Can you work these out from the model? Positions are in its coordinate system, mm. Face numbers are marked on the shaded views. A direction names the side the tool comes from. Give positions to 0.01 mm unless a question says otherwise; leave off trailing zeros. Order: outer loops, then holes, each group sorted by start corner. A loop starts at its lowest first (then second) coordinate and runs counter-clockwise, first axis right, second up. Notation, with made-up numbers: M 84,-1 L 111,-1 A21 ccw 111,31 Z; hole C 41,15.5 d10. An arc over 180 degrees is marked long. Write each question's results on one line, items separated by ' | '.
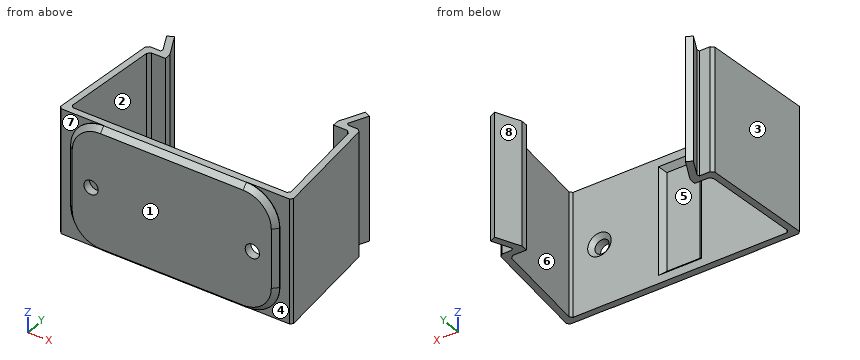
from build123d import *
from OCP.BRepFilletAPI import BRepFilletAPI_MakeChamfer

# Parameters (mm, degrees)
BOSS_EXTRUDE1_DEPTH                               = 38
SKETCH5_W                                         = 63
SKETCH5_H                                         = 38
BOSS_EXTRUDE2_DEPTH                               = 1.6
SKETCH9_W                                         = 10
SKETCH9_H                                         = 30
CUT_EXTRUDE4_DEPTH                                = 1.5
CHAMFER4_SIZE                                     = 1.5
CHAMFER6_SIZE                                     = 0.8
CHAMFER6_SIZE2                                    = 0.738449877
CHAMFER7_SIZE                                     = 0.8
CHAMFER7_SIZE2                                    = 0.880050294
CHAMFER7_SIZE2_2                                  = 0.59857957
CSK_FOR_6_FLAT_HEAD_MACHINE_SCREW_100_D           = 4.3053
CSK_FOR_6_FLAT_HEAD_MACHINE_SCREW_100_DEPTH       = 3.6
CSK_FOR_6_FLAT_HEAD_MACHINE_SCREW_100_CSINK_D     = 7.0866
CSK_FOR_6_FLAT_HEAD_MACHINE_SCREW_100_CSINK_ANGLE = 100
FILLET1_R                                         = 10
CHAMFER10_SIZE                                    = 1.5


with BuildPart() as part:
    # Sketch1 → Boss-Extrude1 (new body)
    with BuildSketch(Plane.XY):
        Polygon((-32.16425811, 32.5), (-27.555232111, 32.5), (-30.546782223, 38.65618727), (-28.747926936, 39.530326652), (-25.331595762, 32.5), (-25.331595762, 30.5), (-30.331595762, 30.5), (-33, 0), (0, 0), (33, 0), (30.331595762, 30.5), (25.331595762, 30.5), (25.331595762, 32.5), (28.747926936, 39.530326652), (30.546782223, 38.65618727), (27.555232111, 32.5), (32.16425811, 32.5), (35.182617002, -2), (0, -2), (-35.182617002, -2), align=None)
    extrude(amount=BOSS_EXTRUDE1_DEPTH)

    # Sketch5 → Boss-Extrude2 (add)
    with BuildSketch(Plane.XZ.offset(2)):
        with Locations((0, 19)):
            Rectangle(SKETCH5_W, SKETCH5_H)
    extrude(amount=BOSS_EXTRUDE2_DEPTH)

    # Sketch9 → Cut-Extrude4 (cut)
    with BuildSketch(Plane(origin=(0, 0, 0), x_dir=(1, 0, 0), z_dir=(0, 1, 0))):
        with Locations((0, -19)):
            Rectangle(SKETCH9_W, SKETCH9_H)
    extrude(amount=-CUT_EXTRUDE4_DEPTH, mode=Mode.SUBTRACT)

    # Chamfer4
    chamfer4_edges = [part.edges().sort_by_distance(p)[0] for p in [
        (0, 0, 34),
        (-5, 0, 19),
        (0, 0, 4),
        (5, 0, 19),
    ]]
    chamfer(chamfer4_edges, length=CHAMFER4_SIZE - 0.0001)  # a hair under: the kernel refuses the full size

    # Chamfer6: one chamfer whose edges measure the first distance from different faces: ONE call of the kernel's chamfer builder (chamfer() names one face for all edges)
    chamfer6_edges_1 = [part.edges().sort_by_distance(p)[0] for p in [
        (-33, 0, 19),
    ]]
    chamfer6_side_1 = [part.faces().sort_by_distance(p)[0] for p in [
        (0, 0, 36.261477311),
    ]]
    chamfer6_edges_2 = [part.edges().sort_by_distance(p)[0] for p in [
        (33, 0, 19),
    ]]
    chamfer6_side_2 = [part.faces().sort_by_distance(p)[0] for p in [
        (31.665797881, 15.25, 19),
    ]]
    chamfer6_edges_3 = [part.edges().sort_by_distance(p)[0] for p in [
        (35.182617002, -2, 19),
    ]]
    chamfer6_side_3 = [part.faces().sort_by_distance(p)[0] for p in [
        (33.341308501, -2, 19),
    ]]
    chamfer6_edges_4 = [part.edges().sort_by_distance(p)[0] for p in [
        (-35.182617002, -2, 19),
    ]]
    chamfer6_side_4 = [part.faces().sort_by_distance(p)[0] for p in [
        (-33.673437556, 15.25, 19),
    ]]
    chamfer6 = BRepFilletAPI_MakeChamfer(part.part.solid().wrapped)
    for e in chamfer6_edges_1:
        chamfer6.Add(CHAMFER6_SIZE, CHAMFER6_SIZE2, e.wrapped, chamfer6_side_1[0].wrapped)  # the first distance lies on this face
    for e in chamfer6_edges_2:
        chamfer6.Add(CHAMFER6_SIZE, CHAMFER6_SIZE2, e.wrapped, chamfer6_side_2[0].wrapped)  # the first distance lies on this face
    for e in chamfer6_edges_3:
        chamfer6.Add(CHAMFER6_SIZE, CHAMFER6_SIZE2, e.wrapped, chamfer6_side_3[0].wrapped)  # the first distance lies on this face
    for e in chamfer6_edges_4:
        chamfer6.Add(CHAMFER6_SIZE, CHAMFER6_SIZE2, e.wrapped, chamfer6_side_4[0].wrapped)  # the first distance lies on this face
    add(Compound.cast(chamfer6.Shape()), mode=Mode.REPLACE)

    # Chamfer7: one chamfer whose edges measure the first distance from different faces: ONE call of the kernel's chamfer builder (chamfer() names one face for all edges)
    chamfer7_edges_1 = [part.edges().sort_by_distance(p)[0] for p in [
        (-30.331595762, 30.5, 19),
    ]]
    chamfer7_side_1 = [part.faces().sort_by_distance(p)[0] for p in [
        (-31.633617807, 15.617819926, 19),
    ]]
    chamfer7_edges_2 = [part.edges().sort_by_distance(p)[0] for p in [
        (30.331595762, 30.5, 19),
    ]]
    chamfer7_side_2 = [part.faces().sort_by_distance(p)[0] for p in [
        (27.831595762, 30.5, 19),
    ]]
    chamfer7_edges_3 = [part.edges().sort_by_distance(p)[0] for p in [
        (27.555232111, 32.5, 19),
    ]]
    chamfer7_side_3 = [part.faces().sort_by_distance(p)[0] for p in [
        (29.859745111, 32.5, 19),
    ]]
    chamfer7_edges_4 = [part.edges().sort_by_distance(p)[0] for p in [
        (32.16425811, 32.5, 19),
    ]]
    chamfer7_side_4 = [part.faces().sort_by_distance(p)[0] for p in [
        (33.641257483, 15.617819926, 19),
    ]]
    chamfer7_edges_5 = [part.edges().sort_by_distance(p)[0] for p in [
        (-32.16425811, 32.5, 19),
    ]]
    chamfer7_side_5 = [part.faces().sort_by_distance(p)[0] for p in [
        (-29.859745111, 32.5, 19),
    ]]
    chamfer7_edges_6 = [part.edges().sort_by_distance(p)[0] for p in [
        (-27.555232111, 32.5, 19),
    ]]
    chamfer7_side_6 = [part.faces().sort_by_distance(p)[0] for p in [
        (-29.051007167, 35.578093635, 19),
    ]]
    chamfer7 = BRepFilletAPI_MakeChamfer(part.part.solid().wrapped)
    for e in chamfer7_edges_1:
        chamfer7.Add(CHAMFER7_SIZE, CHAMFER7_SIZE2, e.wrapped, chamfer7_side_1[0].wrapped)  # the first distance lies on this face
    for e in chamfer7_edges_2:
        chamfer7.Add(CHAMFER7_SIZE, CHAMFER7_SIZE2, e.wrapped, chamfer7_side_2[0].wrapped)  # the first distance lies on this face
    for e in chamfer7_edges_3:
        chamfer7.Add(CHAMFER7_SIZE, CHAMFER7_SIZE2_2, e.wrapped, chamfer7_side_3[0].wrapped)  # the first distance lies on this face
    for e in chamfer7_edges_4:
        chamfer7.Add(CHAMFER7_SIZE, CHAMFER7_SIZE2, e.wrapped, chamfer7_side_4[0].wrapped)  # the first distance lies on this face
    for e in chamfer7_edges_5:
        chamfer7.Add(CHAMFER7_SIZE, CHAMFER7_SIZE2, e.wrapped, chamfer7_side_5[0].wrapped)  # the first distance lies on this face
    for e in chamfer7_edges_6:
        chamfer7.Add(CHAMFER7_SIZE, CHAMFER7_SIZE2_2, e.wrapped, chamfer7_side_6[0].wrapped)  # the first distance lies on this face
    add(Compound.cast(chamfer7.Shape()), mode=Mode.REPLACE)

    # CSK for #6 Flat Head Machine Screw (100)1
    with Locations(Plane(origin=(0, 0, 0), x_dir=(1, 0, 0), z_dir=(0, 1, 0))):
        with Locations((24.3, -19), (-24.3, -19)):
            CounterSinkHole(CSK_FOR_6_FLAT_HEAD_MACHINE_SCREW_100_D / 2, CSK_FOR_6_FLAT_HEAD_MACHINE_SCREW_100_CSINK_D / 2, depth=CSK_FOR_6_FLAT_HEAD_MACHINE_SCREW_100_DEPTH, counter_sink_angle=CSK_FOR_6_FLAT_HEAD_MACHINE_SCREW_100_CSINK_ANGLE)

    # Fillet1
    fillet1_edges = [part.edges().sort_by_distance(p)[0] for p in [
        (-31.5, -2.8, 0),
        (31.5, -2.8, 0),
        (31.5, -2.8, 38),
        (-31.5, -2.8, 38),
    ]]
    fillet(fillet1_edges, radius=FILLET1_R)

    # Chamfer10
    chamfer10_edges = [part.edges().sort_by_distance(p)[0] for p in [
        (-31.5, -3.6, 19),
        (0, -3.6, 38),
        (0, -3.6, 0),
        (31.5, -3.6, 19),
        (28.571067812, -3.6, 35.071067812),
        (28.571067812, -3.6, 2.928932188),
        (-28.571067812, -3.6, 2.928932188),
        (-28.571067812, -3.6, 35.071067812),
    ]]
    chamfer(chamfer10_edges, length=CHAMFER10_SIZE)


solid = part.part
(1) Imagine slicing it at B-B, the plane y = 4.5. Write out the boundary of the cut face in (x, z), plus the area to 3 significant figures.
Data:
outline: M -34.61,0 L -32.61,0 L -32.61,38 L -34.61,38 Z; M 32.61,0 L 34.61,0 L 34.61,38 L 32.61,38 Z | area: 153 mm2
(2) I need wall thicknesses on L1, parallel to Z at x = -24.3, y = -1.95; L2, parallel to Y at x = 2, z = 12; L3, parallel to Y at x = 8.5, z = 9.5. Which ranges of each line are inside material? Lowest first, please. Write a range as from..to.
Data:
L1: z = 0..16.85, 21.15..38 | L2: y = -3.6..-1.5 | L3: y = -3.6..0
(3) Will these pins go through, and if not, where does the flat tip stop? P1, Ø4, axis at x = -6, z = 28.5, coming from the +Y side; P2, Ø12, axis at y = 20.5, z = 10.5, coming from the -X side; P3, Ø3.5, axis at x = -29.5, z = 10.5, coming from the +Y side; P4, Ø2, axis at y = 31.5, z = 18, coming from the -X side.
Data:
P1: stops at y = 0 | P2: stops at x = -33.74 | P3: stops at y = 39.53 | P4: stops at x = -32.34
(4) Imagine slicing it at D-D, the plane y = 35. Write out the boundary of the cut face in (x, z), plus the area to 3 significant figures.
Data:
outline: M -28.77,0 L -26.55,0 L -26.55,38 L -28.77,38 Z; M 26.55,0 L 28.77,0 L 28.77,38 L 26.55,38 Z | area: 169 mm2
(5) For the marked faces 1, 2, 3, 4 and 5, which set-ups out of +Z, -Z, +X, -X, +Y, -Y let a thin tool reach every point of the face, with its end or its side?
Data:
face 1: +Z, -Z, +X, -X, -Y | face 2: +Z, -Z | face 3: +Z, -Z, -X, +Y | face 4: +X, -Y | face 5: +Y
(6) We'd pull the mould along Y, two halves only. Please class the marked faces 6, 7 and 8: +Y half, -Y half, draft (parallel to the pull), parting line (faces both ways), or undercut.
Data:
face 6: undercut | face 7: -Y half | face 8: +Y half
(7) Imagine slicing it at C-C, the plane z = 19. Count the separate pieces of the cut face and the enclosed holes in it, plus the area to 3 significant figures.
Data:
separate pieces: 3 | enclosed holes: 0 | area: 367 mm2
